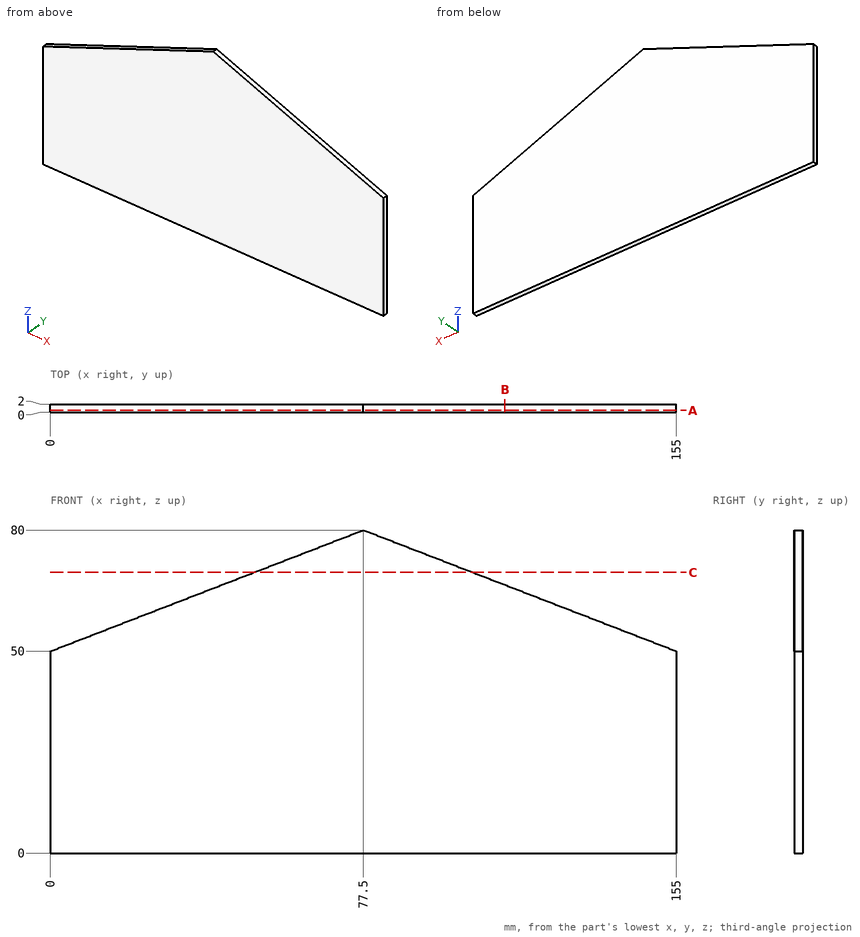
Geometry check sheet. Reference: drawing and pictorial views, mm from the part's lowest x, y, z. Round coordinates to 2 decimals unless told otherwise and drop trailing zeros. Order: outer loops, then holes, each group sorted by start corner. A loop starts at its lowest first (then second) coordinate and runs counter-clockwise, first axis right, second up.
Q1. Cross-section at B-B, the plane x = 112.5. Enter the section's corners in (y, z), plus the area to 3 significant figures.
Filled sheet:
outline: (0, 0) - (2, 0) - (2, 66.45) - (0, 66.45) - close
area: 133 mm2
Q2. Scan lines: L1, parallel to Z at x = 8, y = 0.45; L2, parallel to Z at x = 105.5, y = 1.7. Record each from-to range of solid material in increasing order.
Filled sheet:
L1: z = 0 to 53.1
L2: z = 0 to 69.16
Q3. Cross-section at A-A, the plane y = 0.45. Enter the section's corners in (x, z), plus the area to 3 significant figures.
Filled sheet:
outline: (0, 0) - (155, 0) - (155, 50) - (77.5, 80) - (0, 50) - close
area: 10,100 mm2
Q4. Cross-section at C-C, the plane z = 69.5. Enter the section's corners in (x, y) (3 decimals).
Filled sheet:
outline: (50.375, 0) - (104.625, 0) - (104.625, 2) - (50.375, 2) - close
